Here's how the part is built. I have some questions about the finished solid (model axes, mm). A direction names the side the tool comes from. Round coordinates to 2 decimals unless told otherwise and drop trailing zeros. Loops run counter-clockwise (first coordinate to the right, second up) from the corner with the lowest first, then second, coordinate; pieces in that order, holes last. Notation, with made-up numbers: M -27.75,49.5 L 12.25,49.5 A17 cw 12.25,76.5 Z; hole C 37,-9 d3. An arc over 180 degrees is marked long. Use a Markdown table: item, result.
Autodesk Inventor part; units mm, degrees
ref_plane "Work Plane1" through (0, 0, 15) normal (0, 0, 1) x (1, 0, 0)
ref_plane "YZ Plane" through (0, 0, 0) normal (1, 0, 0) x (0, 1, 0)
ref_plane "XZ Plane" through (0, 0, 0) normal (0, 1, 0) x (-1, 0, 0)
sketch "Sketch1" plane through (0, 0, 0) normal (0, 0, 1) x (1, 0, 0)
  line L0 (-10, 40) -> (-10, 0)
  line L1 (-10, 0) -> (0, 0)
  line L2 (0, 0) -> (9.5, 5)
  line L3 (9.5, 5) -> (9.5, 40)
  line L4 (9.5, 40) -> (-10, 40)
  dimension "d0" = 40
  dimension "d2" = 10
  dimension "d55" = 9.5
  dimension "d57" = 35
extrude "Extrusion1" add sketch "Sketch1" along normal mid plane 35
ref_plane "Work Plane1" through (0, 0, 15) normal (0, 0, 1) x (1, 0, 0)
sketch "Sketch2" plane through (0, 0, 15) normal (0, 0, 1) x (1, 0, 0)
  line L0 (-10, 40) -> (-10, 0)
  line L1 (-10, 0) -> (0, 0)
  line L2 (-10, 0) -> (-31, 0)
  line L3 (-10, 0) -> (11, 0) construction
  line L4 (0, 0) -> (9.5, 5)
  line L5 (9.5, 5) -> (9.5, 40)
  line L6 (9.5, 40) -> (-10, 40)
  line L7 (-31, 0) -> (-10, 25)
  line L8 (-10, 0) -> (-10, 25)
  dimension "d9" = 21
  dimension "d10" = 180
  dimension "d88" = 25
extrude "Extrusion2" add sketch "Sketch2" along normal mid plane 3 contours L0 L2 L7
mirror "Mirror1" about plane through (0, 0, 0) normal (0, 0, 1) of "Extrusion2"
sketch "Sketch3" plane through (-10, 0, 17.5) normal (0, -1, 0) x (1, 0, 0)
  line L0 (-40, 2) -> (-15.2727, 11)
  line L1 (-15.2727, 11) -> (10, 11)
  line L2 (10, 11) -> (10, -46)
  line L3 (-40, 2) -> (-40, -37)
  line L4 (-40, -37) -> (-15.2727, -46)
  line L5 (-15.2727, -46) -> (10, -46)
  line L6 (10, -35) -> (10, 0)
  line L7 (10, -35) -> (10, 0)
  line L8 (0, 0) -> (0, -1)
  line L9 (10, -35) -> (0, -35)
  line L10 (0, 0) -> (10, 0)
  line L11 (-21, -1) -> (0, -1)
  line L12 (-21, -4) -> (-21, -1)
  line L13 (0, -4) -> (-21, -4)
  line L14 (0, -4) -> (0, -31)
  line L15 (0, -31) -> (-21, -31)
  line L16 (-21, -31) -> (-21, -34)
  line L17 (-21, -34) -> (0, -34)
  line L18 (0, -34) -> (0, -35)
  point P0 (10, -17.5)
  point P1 (-2.6364, 11)
  point P2 (10, -17.5)
  point P3 (10, -17.5)
  point P4 (10, -17.5)
  point P5 (-2.6364, -46)
  point P6 (-40, -17.5)
  point P7 (10, -17.5)
  point P8 (10, -35)
  point P9 (10, 0)
  dimension "d17" = 57
  dimension "d18" = 39
  dimension "d19" = 9
  dimension "d20" = 9
  dimension "d21" = 50
  dimension "d76" = 110
extrude "Extrusion3" add sketch "Sketch3" along normal blind 15
sketch "Sketch4" plane through (-10, 0, 17.5) normal (0, 1, 0) x (1, 0, 0)
  line L0 (10, 17.5) -> (-48, 17.5) construction
  line L1 (-32, 10) -> (-12, 10) construction
  line L2 (-32, 25) -> (-32, 10) construction
  line L3 (10, 35) -> (0, 35)
  line L4 (10, 46) -> (10, 35)
  line L5 (-15.2727, 46) -> (10, 46)
  line L6 (-40, 37) -> (-15.2727, 46)
  line L7 (-40, -2) -> (-40, 37)
  line L8 (-15.2727, -11) -> (-40, -2)
  line L9 (10, -11) -> (-15.2727, -11)
  line L10 (10, 0) -> (10, -11)
  line L11 (0, 0) -> (10, 0)
  line L12 (0, 0) -> (0, 1)
  line L13 (-21, 1) -> (0, 1)
  line L14 (-21, 4) -> (-21, 1)
  line L15 (0, 4) -> (-21, 4)
  line L16 (0, 4) -> (0, 31)
  line L17 (0, 31) -> (-21, 31)
  line L18 (-21, 31) -> (-21, 34)
  line L19 (-21, 34) -> (0, 34)
  line L20 (0, 34) -> (0, 35)
  point P0 (-32, 17.5)
  point P1 (-19, 17.5)
  dimension "d26" = 20
  dimension "d27" = 15
  dimension "d58" = 13
  dimension "d59" = 8
hole "Hole1" at (-42, 0, 7.5) at (-22, 0, 7.5) at (-42, 0, -7.5) direction (0, -1, 0) diameter 3.1 end through all
sketch "Sketch5" plane through (0, 0, -17.5) normal (1, 0, 0) x (0, 0, -1)
  line L0 (11, 0) -> (0, 0)
  line L1 (-35, 0) -> (-46, 0)
  line L2 (-46, 0) -> (-46, -15)
  line L3 (11, -15) -> (-46, -15)
  line L4 (11, 0) -> (11, -15)
  line L5 (-46, 0) -> (-46, -15)
  line L6 (-21, -4) -> (9, -4)
  line L7 (9, -4) -> (9, -14)
  line L8 (9, -14) -> (-21, -14)
  line L9 (-21, -14) -> (-21, -4)
  line L10 (0, 0) -> (-35, 0)
  point P0 (-17.5, 0)
  point P1 (-17.5, 0)
  point P2 (-46, -7.5)
  point P3 (-46, -7.5)
  point P4 (11, -12.5)
  point P5 (11, -2.5)
  dimension "d46" = 30
  dimension "d47" = 10
  dimension "d48" = 2
  dimension "d49" = 4
extrude "Extrusion4" cut sketch "Sketch5" against normal blind 30 contours L6 L7 L8 L9
sketch "Sketch6" plane through (-10, 0, 17.5) normal (0, 1, 0) x (1, 0, 0)
  circle A0 centre (-32, 25) radius 1.55
  circle A1 centre (-12, 10) radius 1.55
  circle A2 centre (-32, 10) radius 1.55
  line L0 (10, 35) -> (0, 35)
  line L1 (10, 46) -> (10, 35)
  line L2 (-15.2727, 46) -> (10, 46)
  line L3 (-40, 37) -> (-15.2727, 46)
  line L4 (-40, -2) -> (-40, 37)
  line L5 (-15.2727, -11) -> (-40, -2)
  line L6 (10, -11) -> (-15.2727, -11)
  line L7 (10, 0) -> (10, -11)
  line L8 (0, 0) -> (10, 0)
  line L9 (0, 0) -> (0, 1)
  circle A3 centre (-12, 25) radius 2.9
  line L10 (-21, 1) -> (0, 1)
  line L11 (-21, 4) -> (-21, 1)
  line L12 (0, 4) -> (-21, 4)
  line L13 (0, 4) -> (0, 31)
  line L14 (0, 31) -> (-21, 31)
  line L15 (-21, 31) -> (-21, 34)
  line L16 (-21, 34) -> (0, 34)
  line L17 (0, 34) -> (0, 35)
  point P0 (10, 17.5)
  dimension "d41" = 5.8
  dimension "d42" = 20
  dimension "d43" = 15
extrude "Extrusion5" cut sketch "Sketch6" against normal blind 3 contours A3
sketch "Sketch7" plane through (-10, -15, 17.5) normal (0, -1, 0) x (1, 0, 0)
  circle A0 centre (-12, -25) radius 1.55
  circle A1 centre (-32, -25) radius 1.55
  circle A2 centre (-12, -10) radius 1.55
  circle A3 centre (-32, -10) radius 1.55
  line L0 (10, -46) -> (10, 11)
  line L1 (10, 11) -> (-15.2727, 11)
  line L2 (-15.2727, 11) -> (-40, 2)
  line L3 (-40, 2) -> (-40, -37)
  line L4 (-40, -37) -> (-15.2727, -46)
  line L5 (-15.2727, -46) -> (10, -46)
  point P0 (10, -17.5)
  dimension "d50" = 15
  dimension "d51" = 20
  dimension "d52" = 3.1
extrude "Extrusion6" cut sketch "Sketch7" against normal up to surface (1 mm away) contours A0
sketch "Sketch8" plane through (0, 0, 17.5) normal (0, 0, 1) x (1, 0, 0)
  line L0 (-10, 0) -> (0, 0)
  line L1 (0, 0) -> (9.5, 5)
  line L2 (9.5, 5) -> (9.5, 40)
  line L3 (9.5, 40) -> (-10, 40)
  line L4 (-10, 40) -> (-10, 0)
  line L5 (-10.7901, 28) -> (5, 28) construction
  line L6 (5, 28) -> (5, 11.9362) construction
  line L7 (5, 11.9362) -> (-10.7901, 11.9362) construction
  line L8 (-10.7901, 11.9362) -> (-10.7901, 28) construction
  line L9 (-5.3559, 21.4049) -> (-7.6037, 21.4049)
  line L10 (-7.6037, 21.4049) -> (-7.6037, 17)
  line L11 (-7.6037, 17) -> (-9.555, 17)
  line L12 (-9.555, 17) -> (-9.555, 28)
  line L13 (-9.555, 28) -> (-5.3889, 28)
  spline S0 degree 2 poles (-5.3889, 28) (-4.5326, 28) (-3.207, 27.5389) (-2.3095, 26.7485) (-1.832, 25.637) (-1.832, 24.9783) knots 0 0 0 1 2 3 4 4 4
  line L14 (-1.832, 24.9783) -> (-1.832, 24.4102)
  spline S1 degree 2 poles (-1.832, 24.4102) (-1.832, 23.5457) (-2.6883, 22.1542) (-3.5445, 21.7754) knots 0 0 0 1 2 2 2
  spline S2 degree 2 poles (-3.5445, 21.7754) (-2.9929, 20.5651) (-1.939, 18.2021) (-1.3956, 17) knots 0 0 0 1 2 2 2
  line L15 (-1.3956, 17) -> (-3.5116, 17)
  line L16 (-3.5116, 17) -> (-5.3559, 21.4049)
  line L17 (-7.6037, 26.3698) -> (-7.6037, 23.0434)
  line L18 (-7.6037, 23.0434) -> (-5.8005, 23.0434)
  spline S3 degree 2 poles (-5.8005, 23.0434) (-4.6725, 23.0434) (-3.7751, 23.8338) (-3.7751, 24.4596) knots 0 0 0 1 2 2 2
  line L19 (-3.7751, 24.4596) -> (-3.7751, 24.9207)
  spline S4 degree 2 poles (-3.7751, 24.9207) (-3.7751, 25.5546) (-4.6231, 26.3698) (-5.6359, 26.3698) knots 0 0 0 1 2 2 2
  line L20 (-5.6359, 26.3698) -> (-7.6037, 26.3698)
  line L21 (7.0273, 21.9237) -> (2.4659, 21.9237)
  line L22 (2.4659, 21.9237) -> (2.4659, 17)
  line L23 (2.4659, 17) -> (0.5146, 17)
  line L24 (0.5146, 17) -> (0.5146, 28)
  line L25 (0.5146, 28) -> (2.4659, 28)
  line L26 (2.4659, 28) -> (2.4659, 23.5457)
  line L27 (2.4659, 23.5457) -> (7.0273, 23.5457)
  line L28 (7.0273, 23.5457) -> (7.0273, 28)
  line L29 (7.0273, 28) -> (8.9869, 28)
  line L30 (8.9869, 28) -> (8.9869, 17)
  line L31 (8.9869, 17) -> (7.0273, 17)
  line L32 (7.0273, 17) -> (7.0273, 21.9237)
  point P0 (-7, 15)
  dimension "d68" = 12
  dimension "d69" = 15
extrude "Extrusion7" cut sketch "Sketch8" against normal blind 5 contours L9 L10 L11 L12 L13 S0 L14 S1 S2 L15 L16 | L21 L22 L23 L24 L25 L26 L27 L28 L29 L30 L31 L32
sketch "Sketch9" plane through (0, 0, -17.5) normal (0, 0, -1) x (-1, 0, 0)
  line L0 (-0.5146, 17) -> (-0.5146, 28)
  line L1 (0, 0) -> (10, 0)
  line L2 (10, 0) -> (10, 40)
  line L3 (10, 40) -> (-9.5, 40)
  line L4 (-9.5, 40) -> (-9.5, 5)
  line L5 (-9.5, 5) -> (0, 0)
  line L6 (-7.3088, 28) -> (-3.8059, 28) construction
  line L7 (-3.8059, 28) -> (-3.8059, 25.5662) construction
  line L8 (-3.8059, 25.5662) -> (-7.3088, 25.5662) construction
  line L9 (-7.3088, 25.5662) -> (-7.3088, 28) construction
  line L10 (5.5, 50.4054) -> (5.5, 41.2692)
  line L11 (6.1232, 21.3023) -> (1.0421, 21.3023)
  line L12 (1.0421, 21.3023) -> (1.0421, 16.2212)
  line L13 (1.0421, 16.2212) -> (-0.6353, 16.2212)
  line L14 (-0.6353, 16.2212) -> (-0.6353, 21.3023)
  line L15 (-0.6353, 21.3023) -> (-5.7164, 21.3023)
  line L16 (-5.7164, 21.3023) -> (-5.7164, 22.919)
  line L17 (-5.7164, 22.919) -> (-0.6353, 22.919)
  line L18 (-0.6353, 22.919) -> (-0.6353, 28)
  line L19 (-0.6353, 28) -> (1.0421, 28)
  line L20 (1.0421, 28) -> (1.0421, 22.919)
  line L21 (1.0421, 22.919) -> (6.1232, 22.919)
  line L22 (6.1232, 22.919) -> (6.1232, 21.3023)
  dimension "d72" = 12
  dimension "d73" = 15
extrude "Extrusion8" cut sketch "Sketch9" against normal blind 5 contours L11 L12 L13 L14 L15 L16 L17 L18 L19 L20 L21 L22
sketch "Sketch10" plane through (-10, 0, 17.5) normal (0, 1, 0) x (1, 0, 0)
  line L0 (-39.35, 19.5) -> (-4.65, 19.5)
  circle A0 centre (-32, 25) radius 1.55
  circle A1 centre (-32, 10) radius 1.55
  circle A2 centre (-12, 10) radius 1.55
  circle A3 centre (-32, 25) radius 2.9
  circle A4 centre (-32, 10) radius 2.9
  circle A5 centre (-12, 10) radius 2.9
  point P0 (10, 17.5)
  dimension "d77" = 5.8
  dimension "d78" = 5.8
  dimension "d79" = 5.8
extrude "Extrusion9" cut sketch "Sketch10" against normal blind 10 contours A0 | A1 | A3 | A4 | A5
sketch "Sketch12" plane through (-10, 0, 17.5) normal (0, 1, 0) x (1, 0, 0)
  circle A0 centre (-12, 25) radius 2.9
  circle A1 centre (-12, 25) radius 1.55
  point P0 (10, 17.5)
  dimension "d85" = 3.1
extrude "Extrusion11" cut sketch "Sketch12" against normal blind 4 contours A1
sketch "Sketch13" plane through (-10, 0, 17.5) normal (0, 1, 0) x (1, 0, 0)
  circle A0 centre (-12, 10) radius 2.9
  circle A1 centre (-32, 25) radius 2.9
  circle A2 centre (-32, 10) radius 2.9
  circle A3 centre (-12, 25) radius 2.9
  line L0 (10, 35) -> (0, 35)
  line L1 (10, 46) -> (10, 35)
  line L2 (-15.2727, 46) -> (10, 46)
  line L3 (-40, 37) -> (-15.2727, 46)
  line L4 (-40, -2) -> (-40, 37)
  line L5 (-15.2727, -11) -> (-40, -2)
  line L6 (10, -11) -> (-15.2727, -11)
  line L7 (10, 0) -> (10, -11)
  line L8 (0, 0) -> (10, 0)
  line L9 (0, 0) -> (0, 1)
  line L10 (-21, 1) -> (0, 1)
  line L11 (-21, 4) -> (-21, 1)
  line L12 (0, 4) -> (-21, 4)
  line L13 (0, 4) -> (0, 31)
  line L14 (0, 31) -> (-21, 31)
  line L15 (-21, 31) -> (-21, 34)
  line L16 (-21, 34) -> (0, 34)
  line L17 (0, 34) -> (0, 35)
  line L18 (10, -11) -> (-40, -11)
  line L19 (-40, -11) -> (-40, 0)
  line L20 (-40, 0) -> (10, 0)
  line L21 (10, 0) -> (10, -11)
  line L22 (10, 46) -> (-40, 46)
  line L23 (-40, 46) -> (-40, 35)
  line L24 (-40, 35) -> (10, 35)
  line L25 (10, 35) -> (10, 46)
  point P0 (10, 17.5)
  point P1 (10, 40.5)
  point P2 (-40, 35)
  dimension "d89" = 11
  dimension "d92" = 11
  dimension "d93" = 50
extrude "Extrusion12" cut sketch "Sketch13" against normal blind 30 contours L0 L24 L4 L3 L2 L1 | L20 L8 L7 L6 L5 L4
properties part number "gripper"
1. I need wall thicknesses on probe 1 along X at (y, z) = (-12.1, 7.5); probe 2 along Z at (x, y) = (-42, -11.8); probe 3 along Z at (x, y) = (-22, -3.55). Which ranges of each line are inside material? Lowest first, please. Write a range as from..to.
Answer sheet:
| item | result |
|---|---|
| probe 1 | -50..-43.55, -40.45..-23.55, -20.45..0 |
| probe 2 | -17.5..-9.05, -5.95..5.95, 9.05..17.5 |
| probe 3 | -17.5..-9.05, -5.95..4.6, 10.4..17.5 |
2. Which directions (+Z, -Z, +X, -X, +Y, -Y) give clear straight access to the entire face, cutting with the end or side of a thin tool? Please do faces 1 (the face through (3, 22.919, -15)), 2 (the face through (-30, -9, -7)), 3 (the face through (0, 40, 0)), 4 (the face through (5, 23.546, 15)), 5 (the face through (0, -7, 4)).
Answer sheet:
| item | result |
|---|---|
| face 1 | -Z |
| face 2 | -Z, +X |
| face 3 | +Z, -Z, +X, -X, +Y |
| face 4 | +Z |
| face 5 | +Z, -Z, +X, -Y |
3. We'd pull the mould along Z, two halves only. Please class faces 6 (the face through (-6, 25, 17.5)), 7 (the face through (-40.487, -12.535, -7.836)), 8 (the face through (-4, 21.302, -15)): +Z half, -Z half, draft (parallel to the pull), parting line (faces both ways), or undercut.
Answer sheet:
| item | result |
|---|---|
| face 6 | +Z half |
| face 7 | undercut |
| face 8 | draft |
4. Imagine slicing it at A-A, the plane x = -42. Write out the boundary of the cut face in (y, z), then the cut area to 3 significant figures.
Answer sheet:
| item | result |
|---|---|
| outline | M -15,-17.5 L 0,-17.5 L 0,-10.4 L -10,-10.4 L -10,-9.05 L -15,-9.05 Z; M -15,-5.95 L -10,-5.95 L -10,-4.6 L 0,-4.6 L 0,4.6 L -10,4.6 L -10,5.95 L -15,5.95 Z; M -15,9.05 L -10,9.05 L -10,10.4 L 0,10.4 L 0,17.5 L -15,17.5 Z |
| area | 378 mm2 |
5. For pin 1 Ø4 at (x, z) = (-22, -7.5) entering from +Y; pin 2 Ø2.5 at (x, z) = (-42, 7.5) entering from -Y; pin 3 Ø1.3 at (y, z) = (22.5, -15) entering from -X; pin 4 Ø3.5 at (x, z) = (-22, 7.5) entering from +Y, each with a flat end and sliding along its axis, tell me the tip position at first contact or that it passes through.
Answer sheet:
| item | result |
|---|---|
| pin 1 | y = -3 |
| pin 2 | through |
| pin 3 | x = -12.65 |
| pin 4 | y = -10 |
6. Imagine slicing it at D-D, the plane x = 1.5. Write out the boundary of the cut face in (y, z).
Answer sheet:
| item | result |
|---|---|
| outline | M 0.79,-17.5 L 21.3,-17.5 L 21.3,-12.5 L 22.92,-12.5 L 22.92,-17.5 L 40,-17.5 L 40,17.5 L 28,17.5 L 28,12.5 L 17,12.5 L 17,17.5 L 0.79,17.5 Z |
7. Imagine slicing it at C-C, the plane z = -7.5. State how many separate pieces and enclosed holes the cut face has, then the cut area to 3 significant figures.
Answer sheet:
| item | result |
|---|---|
| separate pieces | 4 |
| enclosed holes | 0 |
| area | 1,110 mm2 |
8. Imagine slicing it at B-B, the plane z = 7.5. Write out the boundary of the cut face in (x, y).
Answer sheet:
| item | result |
|---|---|
| outline | M -50,-15 L -43.55,-15 L -43.55,-10 L -44.9,-10 L -44.9,0 L -50,0 Z; M -40.45,-15 L -23.55,-15 L -23.55,-10 L -24.9,-10 L -24.9,0 L -39.1,0 L -39.1,-10 L -40.45,-10 Z; M -20.45,-15 L 0,-15 L 0,0 L 9.5,5 L 9.5,40 L -10,40 L -10,0 L -19.1,0 L -19.1,-10 L -20.45,-10 Z |
